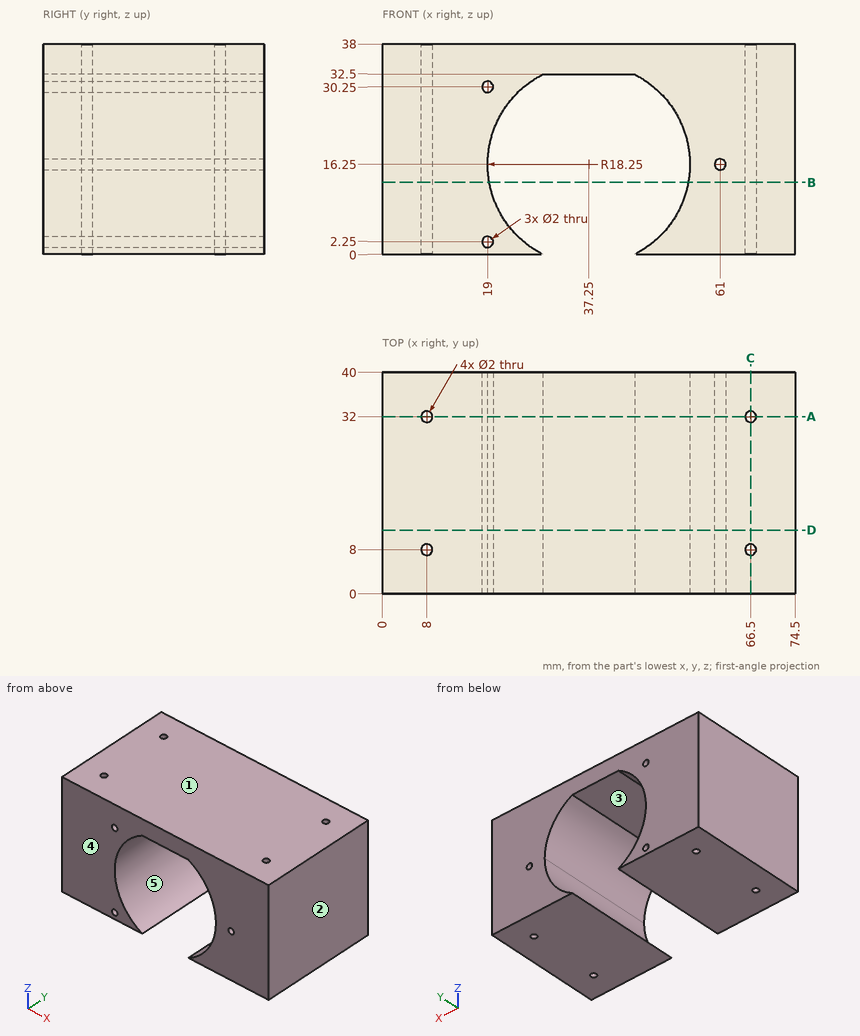
The figure shows three views and two pictorial views of one solid part (mm, origin at its lowest corner). Answer the questions. A direction names the side the tool comes from. Round coordinates to 2 decimals unless told otherwise and drop trailing zeros. Write each loop counter-clockwise with the first axis right and the second up, starting at its lowest first coordinate (ties: lowest second). Pieces come first, ordered by that corner, then holes. Notation, with made-up numbers: M 77.5,-0.5 L 89.5,-0.5 A13 ccw 89.5,4.5 Z; hole C -12,8 d10. An arc over 180 degrees is marked long. Write each question's results on one line, items separated by ' | '. Start each with the question number.
(1) The part is cut by section A-A, the plane y = 32. Write down the section's boundary in (x, z).
(2) This flat-tipped pin is pushed along its axis until it touches: P1, Ø13.5, axis at x = 38.5, y = 28.5, coming from the -Z side. Where does it stop, or does it pass through?
(3) The part is cut by section D-D, the plane y = 11.5. Write down the section's boundary in (x, z).
(4) Find the intervals of material crossed by line 1 (Y direction, x = 66.5, z = 13.5); line 2 (X direction, y = 18, z = 2); line 3 (Z direction, x = 39, y = 13.5), in increasing order.
(5) Determine the mould class of the marked faces 1, 2 and 3 for opening direction X: +X half, -X half, draft (parallel to the pull), parting line (faces both ways), or undercut.
(6) For the marked faces 4 and 5, determine the directions among +Z, -Z, +X, -X, +Y, -Y from which every point of the face is accessible in a straight line to the end or side of a thin tool.
(7) The part is cut by section B-B, the plane z = 13. Write down the section's boundary in (x, y).
(8) The part is cut by section C-C, the plane x = 66.5. Write down the section's boundary in (y, z), and give its area (3 significant figures).
Worked answers:
1) outline: M 0,0 L 7,0 L 7,38 L 0,38 Z; M 9,0 L 28.94,0 A18.25 cw 28.94,32.5 L 45.56,32.5 A18.25 cw 55.5,16.25 A18.25 cw 45.56,0 L 65.5,0 L 65.5,38 L 9,38 Z; M 67.5,0 L 74.5,0 L 74.5,38 L 67.5,38 Z; hole C 19,2.25 d2; hole C 19,30.25 d2; hole C 61,16.25 d2
2) P1: stops at z = 32.5
3) outline: M 0,0 L 28.94,0 A18.25 cw 28.94,32.5 L 45.56,32.5 A18.25 cw 55.5,16.25 A18.25 cw 45.56,0 L 74.5,0 L 74.5,38 L 0,38 Z; hole C 19,2.25 d2; hole C 19,30.25 d2; hole C 61,16.25 d2
4) line 1: y = 0 to 7, 9 to 31, 33 to 40 | line 2: x = 0 to 18.03, 19.97 to 25.85, 48.65 to 74.5 | line 3: z = 32.5 to 38
5) face 1: draft | face 2: +X half | face 3: undercut
6) face 4: +Z, -Z, +X, -X, -Y | face 5: +Y, -Y
7) outline: M 0,0 L 19.29,0 L 19.29,40 L 0,40 Z; M 55.21,0 L 74.5,0 L 74.5,40 L 55.21,40 Z; hole C 8,8 d2; hole C 8,32 d2; hole C 66.5,8 d2; hole C 66.5,32 d2
8) outline: M 0,0 L 7,0 L 7,38 L 0,38 Z; M 9,0 L 31,0 L 31,38 L 9,38 Z; M 33,0 L 40,0 L 40,38 L 33,38 Z | area: 1,370 mm²
